Geometry: see drawing. Coordinates: mm, zero at the bounding-box minimum. A direction names the side the tool comes from. Round coordinates to 2 decimals unless told otherwise and drop trailing zeros. Write each loop counter-clockwise with the first axis right and the second up, starting at its lowest first coordinate (ties: lowest second). Pieces come first, ordered by that corner, then holes. Notation, with made-up numbers: M -21,-10 L 23,-10 A20 ccw 23,22 Z; hole C -34,52.25 d11. An arc over 180 degrees is marked long. Use a Markdown table: item, result.
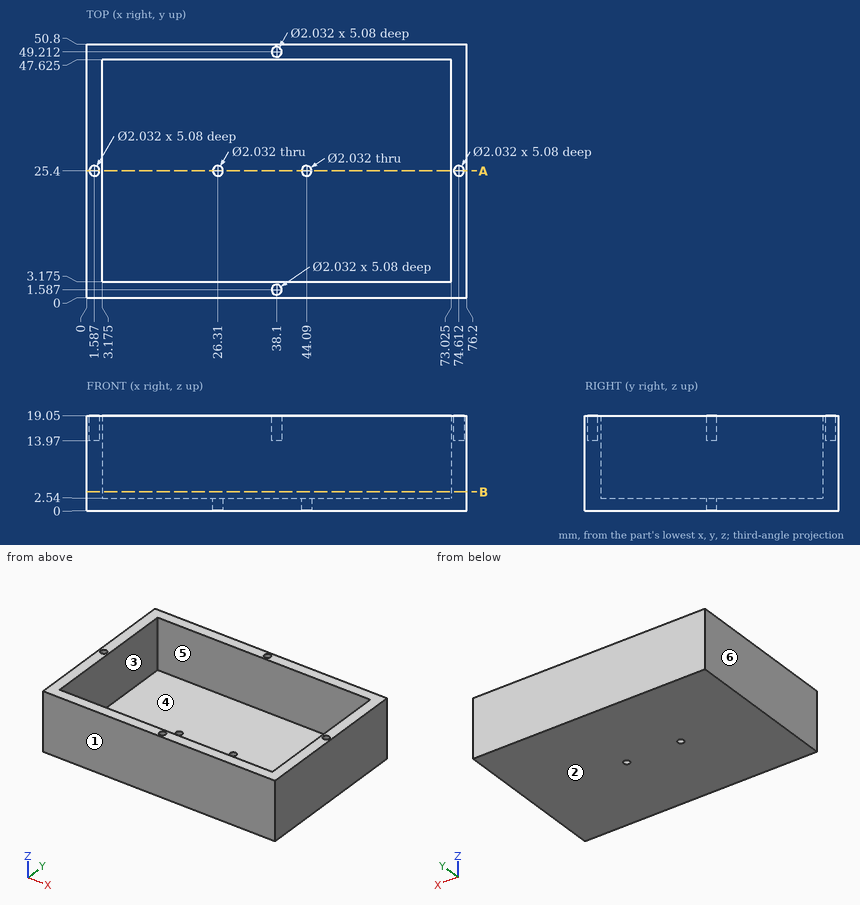
Q1. Reachability of the marked faces 5 and 6 from +Z, -Z, +X, -X, +Y, -Y: full face, straight path, thin tool, end or side. Return the list, or none.
Results are:
| item | result |
|---|---|
| face 5 | +Z |
| face 6 | +Z, -Z, -X, +Y, -Y |
Q2. Section A-A on y = 25.4. Give the number of separate pieces and of enclosed holes in the cut face.
Results are:
| item | result |
|---|---|
| separate pieces | 3 |
| enclosed holes | 0 |
Q3. Section B-B on z = 3.75. Return loops of the section in (x, y) (1 decimal).
Results are:
| item | result |
|---|---|
| outline | M 0,0 L 76.2,0 L 76.2,50.8 L 0,50.8 Z; hole M 3.2,3.2 L 73,3.2 L 73,47.6 L 3.2,47.6 Z |
Q4. Line query: L1, parallel to Y at x = 38.1, z = 18 (1 decimal); L2, parallel to Y at x = 25, z = 17 (1 decimal); L3, parallel to X at y = 28, z = 11.5 (1 decimal). Output: solid intervals per line, ascending.
Results are:
| item | result |
|---|---|
| L1 | 0 to 0.6, 2.6 to 3.2, 47.6 to 48.2, 50.2 to 50.8 |
| L2 | 0 to 3.2, 47.6 to 50.8 |
| L3 | 0 to 3.2, 73 to 76.2 |
Q5. First-contact query: pin 1 Ø1.8 at (x, y) = (38.1, 49.21) entering from +Z; pin 2 Ø3 at (x, y) = (24, 21.5) entering from +Z. Flat tips, straight axial feed; report the tip coordinate or a pass-through.
Results are:
| item | result |
|---|---|
| pin 1 | z = 13.97 |
| pin 2 | z = 2.54 |
Q6. Mould query, pull axis Y, two halves, no side actions, for the marked faces 1, 2, 3 and 4. Classes: +Y half, -Y half, draft (parallel to the pull), parting line (faces both ways), or undercut.
Results are:
| item | result |
|---|---|
| face 1 | -Y half |
| face 2 | draft |
| face 3 | undercut |
| face 4 | undercut |
